Geometry: final body of the model. Coordinates: model frame, mm. A direction names the side the tool comes from. Coordinates: 2 decimals unless noted, no trailing zeros. Loops run counter-clockwise (first coordinate to the right, second up) from the corner with the lowest first, then second, coordinate; pieces in that order, holes last. Notation, with made-up numbers: (39.25, 79.5) -> (65.25, 79.5) arc R11 ccw to (65.25, 90.5) -> close; hole circle Ø7 at (79, -40). An arc over 180 degrees is marked (long way). One line per item, written item: value. Start each with the question number.
Item 1: Section query A-A on z = 0. Return loops of the section in (x, y).
Item 2: Section query B-B on x = 0. Return loops of the section in (y, z).
Item 3: Mould query, pull axis Y, two halves, no side actions, for faces 5 (the cylindrical face through (7.54, -15.92, -36.7)), 6 (the cylindrical face through (7.535, -11.899, -34.958)), 7 (the flat face through (-1.81, -20, -19.14)), 8 (the flat face through (10, -5, -30)). Classes: +Y half, -Y half, draft (parallel to the pull), parting line (faces both ways), or undercut.
Item 4: Set-up query: faces 1 (the flat face through (5, -12.4, -30.9)), 2 (the flat face through (-10, -5, -30)), 3 (the flat face through (-8, -10, -28.05)), 4 (the flat face through (0, 0, -33.05)). Return all of +Z, -Z, +X, -X, +Y, -Y with unobstructed straight access to the full face (end or side cutting, diameter ignored); none if empty.
Item 5: Ray query, probe 1 along X at (y, z) = (-6, 0); probe 2 along X at (y, z) = (-7.5, 5); probe 3 along X at (y, z) = (-1, -28.5). Return the intervals inside material, ascending. Write a range as from..to.
Item 6: Contact query for flat-ended pins moving along their axis: pin 1 Ø5 at (y, z) = (-12, -33.5) entering from +X; pin 2 Ø3.5 at (y, z) = (-12.5, -33.05) entering from -X; pin 3 Ø14 at (y, z) = (-5.5, -29) entering from -X; pin 4 Ø16 at (x, y) = (2.5, 2) entering from -Z. Output: stop coordinate, or through.
Item 7: Section query D-D on z = -24. Return loops of the section in (x, y), then the cut area to 3 significant figures.
Item 8: Section query C-C on y = 3. Return loops of the section in (x, z).
from build123d import *

# Parameters (mm, degrees)
BOSS_EXTRUDE1_DEPTH = 20
BOSS_EXTRUDE2_START = -2.282176
SKETCH2_W           = 20
SKETCH2_H           = 15
BOSS_EXTRUDE2_DEPTH = 12.282176
SKETCH3_R           = 2
BOSS_EXTRUDE3_DEPTH = 5


with BuildPart() as part:
    # Sketch1 → Boss-Extrude1 (new body, symmetric)
    with BuildSketch(Plane(origin=(0, 0, 0), x_dir=(1, 0, 0), z_dir=(0, 1, 0))):
        with BuildLine():
            Line((-11.076364599, -20.214268408), (11.076364599, -20.214268408))
            ThreePointArc((11.076364599, -20.214268408), (0, 23.05), (-11.076364599, -20.214268408))
        make_face()
        with BuildLine():
            Line((-10, -16.214268408), (10, -16.214268408))
            ThreePointArc((10, -16.214268408), (0, 19.05), (-10, -16.214268408))
        make_face(mode=Mode.SUBTRACT)
    extrude(amount=BOSS_EXTRUDE1_DEPTH, both=True)

    # Sketch2 → Boss-Extrude2 (add)
    with BuildSketch(Plane(origin=(0, 0, -23.05), x_dir=(-1, 0, 0), z_dir=(0, 0, -1)).offset(BOSS_EXTRUDE2_START)):
        Rectangle(SKETCH2_W, SKETCH2_H)
    extrude(amount=BOSS_EXTRUDE2_DEPTH)

    # Sketch3 → Boss-Extrude3 (add)
    with BuildSketch(Plane(origin=(10, 0, 0), x_dir=(0, 0, -1), z_dir=(1, 0, 0))):
        with BuildLine():
            Line((28.05, -12.5), (28.05, -7.5))
            Line((28.05, -7.5), (33.05, -7.5))
            ThreePointArc((33.05, -7.5), (36.585533906, -16.035533906), (28.05, -12.5))
        make_face()
        with Locations((33.05, -12.5)):
            Circle(SKETCH3_R, mode=Mode.SUBTRACT)
    boss_extrude3 = extrude(amount=-BOSS_EXTRUDE3_DEPTH)

    # Mirror1: Boss-Extrude3 across plane
    add(boss_extrude3.mirror(Plane(origin=(0, 0, 0), x_dir=(0, 0, 1), z_dir=(1, 0, 0))))


solid = part.part
Reply:
1. outline: (-23.05, -20) -> (-19.05, -20) -> (-19.05, 20) -> (-23.05, 20) -> close; (19.05, -20) -> (23.05, -20) -> (23.05, 20) -> (19.05, 20) -> close
2. outline: (-20, -23.05) -> (-7.5, -23.05) -> (-7.5, -33.05) -> (7.5, -33.05) -> (7.5, -23.05) -> (20, -23.05) -> (20, -19.05) -> (-20, -19.05) -> close; (-20, 16.21) -> (20, 16.21) -> (20, 20.21) -> (-20, 20.21) -> close
3. face 5: parting line
3. face 6: undercut
3. face 7: -Y half
3. face 8: draft
4. face 1: -Z, -Y
4. face 2: -Z, -X, +Y, -Y
4. face 3: +X, -X, -Y
4. face 4: -Z, +X, -X, +Y
5. probe 1: x = -23.05..-19.05, 19.05..23.05
5. probe 2: x = -22.5..-18.38, 18.38..22.5
5. probe 3: x = -10..10
6. pin 1: stops at x = 10
6. pin 2: passes through
6. pin 3: stops at x = -10
6. pin 4: stops at z = -33.05
7. outline: (-10, -7.5) -> (10, -7.5) -> (10, 7.5) -> (-10, 7.5) -> close
7. area: 300 mm²
8. outline: (-11.08, 20.21) arc R23.05 ccw to (-10, -20.77) -> (-10, -33.05) -> (10, -33.05) -> (10, -20.77) arc R23.05 ccw to (11.08, 20.21) -> close; hole (-10, 16.21) arc R19.05 ccw (long way) to (10, 16.21) -> close
